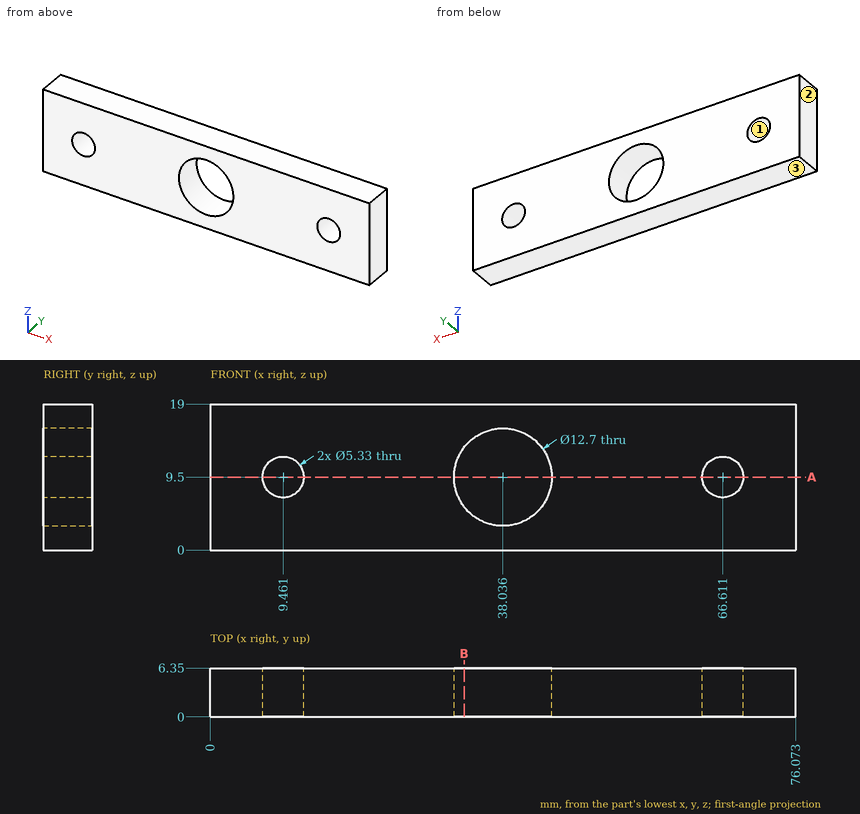
Input: dimensioned drawing with shaded views. Units: mm. Origin: part minimum x, y, z. Coordinates: 2 decimals unless noted, no trailing zeros. Loops run counter-clockwise (first coordinate to the right, second up) from the corner with the lowest first, then second, coordinate; pieces in that order, holes last. Notation, with made-up numbers: (50.5, 76) - (59.5, 76) arc R25 ccw to (59.5, 92) - close; hole circle Ø11 at (53, 37.25). An arc over 180 degrees is marked (long way). One line per question, with ' | ' between items. Start each with the question number.
(1) Draft query along Z for the marked faces 1, 2 and 3. Return one class per face: +Z half, -Z half, draft (parallel to the pull), parting line (faces both ways), or undercut.
(2) Cut plane A-A on z = 9.5. Output: boundary loops of the cut face in (x, y), and give its area (3 significant figures).
(3) First-contact query: pin 1 (10 mm diameter, centred on x = 38.04, z = 9.5, fed in from -Y); pin 2 (8.5 mm diameter, centred on x = 66.61, z = 9.5, fed in from -Y). Flat tips, straight axial feed; report the tip coordinate or a pass-through.
(4) Ray query, L1, parallel to X at y = 5, z = 9.5; L2, parallel to X at y = 6, z = 8.5 (1 decimal); L3, parallel to X at y = 3.75, z = 13.75 (1 decimal). Return the intervals inside material, ascending. Write a range as from..to.
(5) Cut plane B-B on x = 33. Output: boundary loops of the cut face in (y, z).
Here are the results:
1) face 1: undercut | face 2: draft | face 3: -Z half
2) outline: (0, 0) - (6.8, 0) - (6.8, 6.35) - (0, 6.35) - close; (12.13, 0) - (31.69, 0) - (31.69, 6.35) - (12.13, 6.35) - close; (44.39, 0) - (63.95, 0) - (63.95, 6.35) - (44.39, 6.35) - close; (69.28, 0) - (76.07, 0) - (76.07, 6.35) - (69.28, 6.35) - close | area: 335 mm²
3) pin 1: through | pin 2: y = 0
4) L1: 0..6.8, 12.13..31.69, 44.39..63.95, 69.28..76.07 | L2: 0..7, 11.9..31.8, 44.3..64.1, 69.1..76.1 | L3: 0..33.3, 42.8..76.1
5) outline: (0, 0) - (6.35, 0) - (6.35, 5.63) - (0, 5.63) - close; (0, 13.37) - (6.35, 13.37) - (6.35, 19) - (0, 19) - close
